Read the model definition and answer for the solid it produces. Units are mm, in the model's axes. A direction names the side the tool comes from. Coordinates: 2 decimals unless noted, no trailing zeros. Loops run counter-clockwise (first coordinate to the right, second up) from the corner with the lowest first, then second, coordinate; pieces in that order, holes last. Notation, with made-up numbers: (19.5, 31) - (56.5, 31) arc R33 ccw to (56.5, 63) - close; hole circle Ø2 at (-23, -12). An arc over 180 degrees is marked (long way). Use one line per item in the form item = value.
from build123d import *

# Parameters (mm, degrees)
EXTRUDE_1_DEPTH     = 20
CUT_EXTRUDE_1_DEPTH = 1
SKETCH_3_R          = 3.75
SKETCH_3_R_2        = 1.75
EXTRUDE_2_DEPTH     = 1
FILLET_1_R          = 1
CUT_EXTRUDE_2_DEPTH = 1


with BuildPart() as part:
    # 草图1 → 凸台-拉伸1 (new body)
    with BuildSketch(Plane(origin=(0, 0, 0), x_dir=(1, 0, 0), z_dir=(0, 1, 0))):
        Polygon((14.43375673, 0), (7.216878365, 12.5), (-7.216878365, 12.5), (-14.43375673, 0), (-7.216878365, -12.5), (7.216878365, -12.5), align=None)
    extrude(amount=EXTRUDE_1_DEPTH)

    # 草图2 → 切除-拉伸1 (cut)
    with BuildSketch(Plane(origin=(0, 20, 0), x_dir=(1, 0, 0), z_dir=(0, 1, 0))):
        Polygon((5.484827557, -9.5), (10.969655115, 0), (5.484827557, 9.5), (-5.484827557, 9.5), (-10.969655115, 0), (-5.484827557, -9.5), align=None)
    extrude(amount=-CUT_EXTRUDE_1_DEPTH, mode=Mode.SUBTRACT)

    # 草图3 → 凸台-拉伸2 (add)
    # profile 1 of 2: a face of its own
    with BuildSketch(Plane(origin=(0, 19, 0), x_dir=(1, 0, 0), z_dir=(0, 1, 0))):
        with BuildLine():
            Line((8.124640736, -0.490115197), (7.750329512, 2.486441724))
            Line((7.750329512, 2.486441724), (5.47592438, 2.452397232))
            ThreePointArc((5.47592438, 2.452397232), (5.213474627, 2.969794996), (4.902281736, 3.4594268))
            Line((4.902281736, 3.4594268), (6.091552339, 5.39842478))
            Line((6.091552339, 5.39842478), (3.72213075, 7.238490359))
            Line((3.72213075, 7.238490359), (2.137956549, 5.606169975))
            ThreePointArc((2.137956549, 5.606169975), (1.586521082, 5.786445442), (1.02025251, 5.912620808))
            Line((1.02025251, 5.912620808), (0.490115197, 8.124640736))
            Line((0.490115197, 8.124640736), (-2.486441724, 7.750329512))
            Line((-2.486441724, 7.750329512), (-2.452397232, 5.47592438))
            ThreePointArc((-2.452397232, 5.47592438), (-2.969794996, 5.213474627), (-3.4594268, 4.902281736))
            Line((-3.4594268, 4.902281736), (-5.39842478, 6.091552339))
            Line((-5.39842478, 6.091552339), (-7.238490359, 3.72213075))
            Line((-7.238490359, 3.72213075), (-5.606169975, 2.137956549))
            ThreePointArc((-5.606169975, 2.137956549), (-5.786445442, 1.586521082), (-5.912620808, 1.02025251))
            Line((-5.912620808, 1.02025251), (-8.124640736, 0.490115197))
            Line((-8.124640736, 0.490115197), (-7.750329512, -2.486441724))
            Line((-7.750329512, -2.486441724), (-5.47592438, -2.452397232))
            ThreePointArc((-5.47592438, -2.452397232), (-5.213474627, -2.969794996), (-4.902281736, -3.4594268))
            Line((-4.902281736, -3.4594268), (-6.091552339, -5.39842478))
            Line((-6.091552339, -5.39842478), (-3.72213075, -7.238490359))
            Line((-3.72213075, -7.238490359), (-2.137956549, -5.606169975))
            ThreePointArc((-2.137956549, -5.606169975), (-1.586521082, -5.786445442), (-1.02025251, -5.912620808))
            Line((-1.02025251, -5.912620808), (-0.490115197, -8.124640736))
            Line((-0.490115197, -8.124640736), (2.486441724, -7.750329512))
            Line((2.486441724, -7.750329512), (2.452397232, -5.47592438))
            ThreePointArc((2.452397232, -5.47592438), (2.969794996, -5.213474627), (3.4594268, -4.902281736))
            Line((3.4594268, -4.902281736), (5.39842478, -6.091552339))
            Line((5.39842478, -6.091552339), (7.238490359, -3.72213075))
            Line((7.238490359, -3.72213075), (5.606169975, -2.137956549))
            ThreePointArc((5.606169975, -2.137956549), (5.786445442, -1.586521082), (5.912620808, -1.02025251))
            Line((5.912620808, -1.02025251), (8.124640736, -0.490115197))
        make_face()
        with Locations(Location((0, 0, 0), (0, 0, 270))):
            Circle(SKETCH_3_R, mode=Mode.SUBTRACT)
    # profile 2 of 2: a face of its own
    with BuildSketch(Plane(origin=(0, 19, 0), x_dir=(1, 0, 0), z_dir=(0, 1, 0))):
        with Locations(Location((0, 0, 0), (0, 0, 270))):
            Circle(SKETCH_3_R_2)
    extrude(amount=EXTRUDE_2_DEPTH)

    # 圆角1
    fillet_1_edges = [part.edges().sort_by_distance(p)[0] for p in [
        (7.216878365, 10, 12.5),
        (-7.216878365, 10, 12.5),
        (-14.43375673, 10, 0),
        (-7.216878365, 10, -12.5),
        (7.216878365, 10, -12.5),
        (14.43375673, 10, 0),
        (5.484827557, 19.5, 9.5),
        (-5.484827557, 19.5, 9.5),
        (-10.969655115, 19.5, 0),
        (-5.484827557, 19.5, -9.5),
        (5.484827557, 19.5, -9.5),
        (10.969655115, 19.5, 0),
    ]]
    fillet(fillet_1_edges, radius=FILLET_1_R)

    # 草图5 → 切除-拉伸2 (cut)
    with BuildSketch(Plane(origin=(-10.825317547, 0, -6.25), x_dir=(-0.4999999999999999, 0, 0.8660254037844386), z_dir=(-0.8660254037844387, 0, -0.49999999999999994))):
        with BuildLine():
            Line((3.182453488, 16.969587549), (3.182453488, 14.764791287))
            Line((3.182453488, 14.764791287), (-0.912168142, 14.764791287))
            Line((-0.912168142, 14.764791287), (-0.912168142, 12.424655968))
            add(Edge.make_bspline(
                [(-0.912168142, 12.424655968), (-0.847309657, 12.498399491), (-0.720214162, 12.642905944), (-0.505577598, 12.829771532), (-0.281644119, 12.993696487), (-0.03802037, 13.120245746), (0.216657884, 13.221856292), (0.48430812, 13.297309113), (0.76720826, 13.338516205), (0.96030635, 13.344412753), (1.05886066, 13.347422261)],
                knots=[0, 0, 0, 0, 1.045137506, 2.048032268, 3.025244095, 3.994689253, 4.963425262, 5.942900511, 6.950087905, 8, 8, 8, 8], degree=3))
            add(Edge.make_bspline(
                [(1.05886066, 13.347422261), (1.16883757, 13.344864159), (1.382789631, 13.339887557), (1.693785994, 13.307073086), (1.983134795, 13.243970031), (2.252993321, 13.162283164), (2.500375895, 13.052039166), (2.730038976, 12.922999932), (2.933985745, 12.762421538), (3.123965679, 12.581868168), (3.288793274, 12.361712081), (3.431996368, 12.101261287), (3.547683834, 11.794691149), (3.645932383, 11.446555171), (3.720891941, 11.053767841), (3.772768776, 10.617140926), (3.808847597, 10.136794392), (3.811179356, 9.801612815), (3.812395277, 9.626828569)],
                knots=[0, 0, 0, 0, 0.985872992, 1.917944025, 2.797562931, 3.637028488, 4.440265023, 5.220874469, 5.991447987, 6.760933446, 7.563799771, 8.445720104, 9.41645382, 10.49401341, 11.685015475, 12.996358654, 14.433717056, 16, 16, 16, 16], degree=3))
            Line((3.812395277, 9.626828569), (3.812395277, 7.729621071))
            add(Edge.make_bspline(
                [(3.812395277, 7.729621071), (3.811636865, 7.615610244), (3.810174535, 7.39578083), (3.80705838, 7.077408436), (3.793560759, 6.782973949), (3.778578513, 6.511500745), (3.76367309, 6.263371536), (3.737287126, 6.038869904), (3.711892824, 5.837464832), (3.669454906, 5.601271022), (3.597733869, 5.326616934), (3.472868845, 5.012709117), (3.309162628, 4.711425167), (3.108564003, 4.423721493), (2.866599584, 4.157179392), (2.577446527, 3.92540628), (2.24645401, 3.7248973), (1.873113716, 3.557651353), (1.455891936, 3.427693886), (0.995726213, 3.335903519), (0.492669559, 3.279113398), (0.142814297, 3.272028018), (-0.038616051, 3.268353634)],
                knots=[0, 0, 0, 0, 0.989754807, 1.908390848, 2.7635747, 3.547977914, 4.268858805, 4.920711554, 5.509810583, 6.030765573, 7.003130656, 7.968352344, 8.956004724, 9.973318671, 11.006457242, 12.069562088, 13.178372901, 14.357538766, 15.611873537, 16.963616047, 18.425371121, 20, 20, 20, 20], degree=3))
            add(Edge.make_bspline(
                [(-0.038616051, 3.268353634), (-0.243948644, 3.274180091), (-0.644079256, 3.285534078), (-1.226293798, 3.369283972), (-1.771106092, 3.51227482), (-2.196157724, 3.678501355), (-2.511106829, 3.83980469), (-2.728441898, 3.974571457), (-2.926504503, 4.126800061), (-3.108892964, 4.2902182), (-3.271392556, 4.469966225), (-3.421915, 4.658960555), (-3.548207739, 4.867044262), (-3.661278956, 5.089487655), (-3.758939888, 5.334542356), (-3.837250577, 5.608986087), (-3.910253078, 5.912248249), (-3.964865943, 6.247990604), (-4.008619503, 6.61415961), (-4.040877856, 7.010590868), (-4.056594386, 7.437489802), (-4.060074578, 7.732071764), (-4.061877088, 7.884645808)],
                knots=[0, 0, 0, 0, 1.727950145, 3.367247941, 4.937991842, 6.459754912, 7.197724692, 7.914163588, 8.608713051, 9.29788901, 9.972208411, 10.646138941, 11.328189198, 12.016707826, 12.744892405, 13.544369189, 14.416825977, 15.369082158, 16.405235107, 17.52037283, 18.715716525, 20, 20, 20, 20], degree=3))
            Line((-4.061877088, 7.884645808), (-4.061877088, 8.622858842))
            Line((-4.061877088, 8.622858842), (-0.754682694, 8.622858842))
            Line((-0.754682694, 8.622858842), (-0.754682694, 7.766531722))
            add(Edge.make_bspline(
                [(-0.754682694, 7.766531722), (-0.753745858, 7.659902919), (-0.75193704, 7.454026853), (-0.751208911, 7.157043894), (-0.743002222, 6.883906615), (-0.733560957, 6.635339552), (-0.721369171, 6.411380043), (-0.706933178, 6.211159983), (-0.689454556, 6.034806531), (-0.672120944, 5.880501001), (-0.642961084, 5.747231672), (-0.601357722, 5.632643336), (-0.547313566, 5.534055691), (-0.477049795, 5.453064567), (-0.392137997, 5.391956317), (-0.296077191, 5.345048165), (-0.184835288, 5.322009644), (-0.106776695, 5.317852774), (-0.065683863, 5.315664449)],
                knots=[0, 0, 0, 0, 1.823732709, 3.521214749, 5.07892445, 6.496893277, 7.775393918, 8.9147992, 9.929598955, 10.806563962, 11.568882902, 12.256841855, 12.884990135, 13.481481553, 14.073502327, 14.663358483, 15.296344146, 16, 16, 16, 16], degree=3))
            add(Edge.make_bspline(
                [(-0.065683863, 5.315664449), (-0.027731598, 5.317411777), (0.046123876, 5.320812096), (0.149783373, 5.351069232), (0.243322788, 5.398874635), (0.343070554, 5.490110476), (0.439159872, 5.622616497), (0.479320906, 5.768787157), (0.480182252, 5.884957887), (0.487287538, 5.986529514), (0.487850586, 6.126071944), (0.490137715, 6.30324548), (0.496700441, 6.518097802), (0.496919244, 6.770787873), (0.503969738, 7.060282299), (0.504774487, 7.266182326), (0.505200884, 7.375278814)],
                knots=[0, 0, 0, 0, 0.670460052, 1.304721758, 1.895793995, 2.513210904, 3.681360763, 4.748587252, 5.126397419, 5.736946296, 6.550219692, 7.595791071, 8.873918375, 10.355072828, 12.068728984, 14, 14, 14, 14], degree=3))
            Line((0.505200884, 7.375278814), (0.505200884, 10.010699346))
            add(Edge.make_bspline(
                [(0.505200884, 10.010699346), (0.503380579, 10.125575768), (0.500045872, 10.336023509), (0.47546885, 10.622126346), (0.431657196, 10.849379296), (0.366944382, 11.02443971), (0.272609864, 11.14988358), (0.158217982, 11.242089048), (0.013291946, 11.290877165), (-0.089964803, 11.296922757), (-0.144426586, 11.300111446)],
                knots=[0, 0, 0, 0, 1.685864163, 3.088417099, 4.207402662, 5.076902269, 5.799120759, 6.485333904, 7.201103886, 8, 8, 8, 8], degree=3))
            add(Edge.make_bspline(
                [(-0.144426586, 11.300111446), (-0.179832609, 11.298921334), (-0.249105789, 11.296592836), (-0.348784063, 11.271685194), (-0.438878072, 11.228403245), (-0.543268285, 11.155689146), (-0.642858944, 11.044453729), (-0.714660126, 10.910993139), (-0.732507313, 10.774549614), (-0.748399256, 10.626376191), (-0.753089766, 10.428180796), (-0.75411592, 10.279715188), (-0.754682694, 10.197713315)],
                knots=[0, 0, 0, 0, 0.735055358, 1.438162732, 2.117072139, 2.803012647, 4.070557493, 5.191645157, 5.884125613, 6.912400264, 8.294628872, 10, 10, 10, 10], degree=3))
            Line((-0.754682694, 10.197713315), (-4.061877088, 10.197713315))
            Line((-4.061877088, 10.197713315), (-3.904391641, 16.969587549))
            Line((-3.904391641, 16.969587549), (3.182453488, 16.969587549))
        make_face()
    extrude(amount=-CUT_EXTRUDE_2_DEPTH, mode=Mode.SUBTRACT)


solid = part.part
Item 1: For a pull along Y with two mould halves and no side action, classify faces 4 (the flat face through (-10.651, 8.675, -5.566)), 5 (the cylindrical face through (-5.414, 19.493, 9.362)), 6 (the flat face through (-1.9, 20, 3.5)) as +Y half, -Y half, draft (parallel to the pull), parting line (faces both ways), or undercut.
Results below:
face_4 = undercut
face_5 = draft
face_6 = +Y half
Item 2: The part is cut by section C-C on z = -10.5. Give the vertices of the cut face in (x, y).
Results below:
outline = (-8.37, 0) - (8.37, 0) - (8.37, 20) - (-8.37, 20) - close
Item 3: Each of these flat-tipped pins is pushed along its axis until it touches: P1, Ø5, axis at x = 10, y = 14.5, coming from the -Z side; P2, Ø2, axis at y = 15, z = -3, coming from the -X side; P3, Ø2, axis at y = 12, z = -8.5, coming from the -X side. Where does it stop, or does it pass through?
Results below:
P1 = -12.01
P2 = -13.28
P3 = -8.95
Item 4: The part is cut by section A-A on y = 2.5. Give the vertices of the cut face in (x, z).
Results below:
outline = (-14.15, -0.5) - (-7.51, -12) arc R1 ccw to (-6.64, -12.5) - (6.64, -12.5) arc R1 ccw to (7.51, -12) - (14.15, -0.5) arc R1 ccw to (14.15, 0.5) - (7.51, 12) arc R1 ccw to (6.64, 12.5) - (-6.64, 12.5) arc R1 ccw to (-7.51, 12) - (-14.15, 0.5) arc R1 ccw to start
Item 5: Which of the six approach directions +Z, -Z, +X, -X, +Y, -Y give full straight-line access (tool end or side, diameter ignored) to faces 1 (the flat face through (-9.94, 13.61, -6.79)), 2 (the cylindrical face through (7.15, 10.14, 12.36)), 3 (the cylindrical face through (2.96, 19.49, 5.22))?
Results below:
face_1 = -Z
face_2 = +Z, +X, +Y, -Y
face_3 = +Y
Item 6: Find the intervals of material crossed by L1, parallel to X at y = 19.4, z = 0; L2, parallel to Y at x = -9.5, z = 0.25; L3, parallel to Z at x = -7.5, y = 13, in increasing order.
Results below:
L1 = -14.28 to -10.81, -8.06 to -3.75, -1.75 to 1.75, 3.75 to 8.06, 10.81 to 14.28
L2 = 0 to 19
L3 = -12.01 to 12.01
Item 7: The part is cut by section B-B on z = 0. Give the vertices of the cut face in (x, y).
Results below:
outline = (-14.28, 0) - (14.28, 0) - (14.28, 20) - (10.81, 20) - (10.81, 19) - (8.06, 19) - (8.06, 20) - (3.75, 20) - (3.75, 19) - (1.75, 19) - (1.75, 20) - (-1.75, 20) - (-1.75, 19) - (-3.75, 19) - (-3.75, 20) - (-8.06, 20) - (-8.06, 19) - (-10.81, 19) - (-10.81, 20) - (-14.28, 20) - close
